```python
from build123d import *

# Parameters (mm, degrees)
EXTRUDE_1_DEPTH          = 9.45
EXTRUDE_1_DEPTH_BACK     = 9.45
EXTRUDE_2_DEPTH          = 14.45
EXTRUDE_2_DEPTH_BACK     = 14.45
CUT_EXTRUDE_1_DEPTH      = 24.45
CUT_EXTRUDE_1_DEPTH_BACK = 26.45
HOLE_WIZARD_M3_1_D       = 2.5
HOLE_WIZARD_M3_1_DEPTH   = 6.5
HOLE_WIZARD_M3_1_TIP     = 0.751075774


with BuildPart() as part:
    # Sketch 1 → Extrude 1 (new, two sides: drawn at the far end of the back side and taken through both)
    with BuildSketch(Plane(origin=(0, 0, 0), x_dir=(0, 0, -1), z_dir=(1, 0, 0)).offset(-EXTRUDE_1_DEPTH_BACK)):
        Polygon((-10, 7.500004795), (-10, 0.499995205), (-9.500004795, 0), (9.500004795, 0), (10, 0.499995205), (10, 7.500004795), (9.500004795, 8), (4.9, 8), (4.6, 7.7), (-4.6, 7.7), (-4.9, 8), (-9.500004795, 8), align=None)
    extrude(amount=EXTRUDE_1_DEPTH + EXTRUDE_1_DEPTH_BACK)

    # Sketch 2 → Extrude 2 (add, two sides: drawn at the far end of the back side and taken through both)
    with BuildSketch(Plane(origin=(0, 0, 0), x_dir=(0, 0, -1), z_dir=(1, 0, 0)).offset(-EXTRUDE_2_DEPTH_BACK)):
        Polygon((-9.8, 6.70000959), (-9.8, 0.599980104), (-9.200019896, 0), (9.200019896, 0), (9.8, 0.599980104), (9.8, 6.70000959), (8.80000959, 7.7), (-8.80000959, 7.7), align=None)
    extrude(amount=EXTRUDE_2_DEPTH + EXTRUDE_2_DEPTH_BACK)

    # Sketch 3 → Cut-Extrude 1 (cut, two sides: drawn at the far end of the back side and taken through both)
    with BuildSketch(Plane(origin=(0, 0, 0), x_dir=(0, 0, -1), z_dir=(1, 0, 0)).offset(-CUT_EXTRUDE_1_DEPTH_BACK)):
        with BuildLine():
            Line((-4.5, 4.199974593), (-4.5, 3.5583))
            ThreePointArc((-4.5, 3.5583), (-4.475010695, 3.475400506), (-4.408368985, 3.420122355))
            ThreePointArc((-4.408368985, 3.420122355), (-4.141124334, 3.252255308), (-3.93950231, 3.009464023))
            ThreePointArc((-3.93950231, 3.009464023), (-3.898814145, 2.964704671), (-3.843755349, 2.939655613))
            Line((-3.843755349, 2.939655613), (-3.466644651, 2.853644387))
            ThreePointArc((-3.466644651, 2.853644387), (-3.382732565, 2.800932608), (-3.35, 2.7074))
            Line((-3.35, 2.7074), (-3.35, 2.2926))
            ThreePointArc((-3.35, 2.2926), (-3.382732565, 2.199067392), (-3.466644651, 2.146355613))
            Line((-3.466644651, 2.146355613), (-3.843755349, 2.060344387))
            ThreePointArc((-3.843755349, 2.060344387), (-3.898814145, 2.035295329), (-3.93950231, 1.990535977))
            ThreePointArc((-3.93950231, 1.990535977), (-4.141123452, 1.74774336), (-4.408368985, 1.579877645))
            ThreePointArc((-4.408368985, 1.579877645), (-4.475010695, 1.524599494), (-4.5, 1.4417))
            Line((-4.5, 1.4417), (-4.5, -1.500004795))
            Line((-4.5, -1.500004795), (-4.000004795, -2))
            Line((-4.000004795, -2), (1.4, -2))
            ThreePointArc((1.4, -2), (1.8, -1.8), (2.2, -2))
            Line((2.2, -2), (4.000004795, -2))
            Line((4.000004795, -2), (4.5, -1.500004795))
            Line((4.5, -1.500004795), (4.5, 1.4417))
            ThreePointArc((4.5, 1.4417), (4.475010695, 1.524599494), (4.408368985, 1.579877645))
            ThreePointArc((4.408368985, 1.579877645), (4.141124334, 1.747744692), (3.93950231, 1.990535977))
            ThreePointArc((3.93950231, 1.990535977), (3.898814145, 2.035295329), (3.843755349, 2.060344387))
            Line((3.843755349, 2.060344387), (3.466644651, 2.146355613))
            ThreePointArc((3.466644651, 2.146355613), (3.382732565, 2.199067392), (3.35, 2.2926))
            Line((3.35, 2.2926), (3.35, 2.7074))
            ThreePointArc((3.35, 2.7074), (3.382732565, 2.800932608), (3.466644651, 2.853644387))
            Line((3.466644651, 2.853644387), (3.843755349, 2.939655613))
            ThreePointArc((3.843755349, 2.939655613), (3.898814145, 2.964704671), (3.93950231, 3.009464023))
            ThreePointArc((3.93950231, 3.009464023), (4.141123452, 3.25225664), (4.408368985, 3.420122355))
            ThreePointArc((4.408368985, 3.420122355), (4.475010695, 3.475400506), (4.5, 3.5583))
            Line((4.5, 3.5583), (4.5, 4.199974593))
            Line((4.5, 4.199974593), (4.199974593, 4.5))
            Line((4.199974593, 4.5), (-4.199974593, 4.5))
            Line((-4.199974593, 4.5), (-4.5, 4.199974593))
        make_face()
    extrude(amount=CUT_EXTRUDE_1_DEPTH + CUT_EXTRUDE_1_DEPTH_BACK, mode=Mode.SUBTRACT)

    # Sketch 12 → Cut-Revolve 6 (revolve, cut)
    with BuildSketch(Plane.XY.offset(5), mode=Mode.PRIVATE) as cut_revolve_6_sk:
        Polygon((-13.45, 6.2), (-13.45, 7), (-13.2605, 6.8105), (-9.45, 6.8105), (-9.097527661, 6.2), align=None)
    revolve(cut_revolve_6_sk.sketch.rotate(Axis((-9.097527661, 6.2, 5), (-1, 0, 0)), 270), axis=Axis((-9.097527661, 6.2, 5), (-1, 0, 0)), mode=Mode.SUBTRACT)

    # Hole Wizard M3 _1
    with Locations(Plane(origin=(0, 8, 0), x_dir=(1, 0, 0), z_dir=(0, 1, 0))):
        with Locations((5, -7.5), (-5, -7.5), (5, 7.5), (-5, 7.5)):
            Hole(HOLE_WIZARD_M3_1_D / 2, depth=HOLE_WIZARD_M3_1_DEPTH)
            with Locations((0, 0, -(HOLE_WIZARD_M3_1_DEPTH + HOLE_WIZARD_M3_1_TIP / 2))):  # 118° drill point
                Cone(0, HOLE_WIZARD_M3_1_D / 2, HOLE_WIZARD_M3_1_TIP, mode=Mode.SUBTRACT)


solid = part.part
```
Source: CAD feature listing. Evaluate the final solid. Frame: model axes, mm. A direction names the side the tool comes from. Give positions to 0.01 mm unless a question says otherwise; leave off trailing zeros. Order: outer loops, then holes, each group sorted by start corner. A loop starts at its lowest first (then second) coordinate and runs counter-clockwise, first axis right, second up.
(1) Pull-direction query (X, two-part tool) for faces 1 (the face through (5.27, 4.7, 8.72)), 2 (the face through (-14.45, 5, 0)), 3 (the face through (12, 4, -9.8)), 4 (the face through (4.78, 0.88, -7.51)); classes: +X half, -X half, draft (parallel to the pull), parting line (faces both ways), or undercut.
(2) Section query A-A (y = 5). Return the cut outline in (x, z), plus the area to 3 significant figures.
(3) Contact query for flat-ended pins moving along their axis: P1, Ø4, axis at x = -12, y = 3.5, coming from the +Z side; P2, Ø2, axis at x = 5, z = -7.5, coming from the +Y side; P3, Ø1.5, axis at x = 13, y = 3.5, coming from the -Z side. Output: stop coordinate, or through.
(4) Access query for faces 5 (the face through (-11.329, 5.829, 4.516)), 6 (the face through (12, 4, 9.8)), 7 (the face through (0, 4.5, 0)). Directions: +Z, -Z, +X, -X, +Y, -Y. A direction counts if a zero-diameter tool reaches every point of the face in a straight line with its end or side. Return the directions, or none.
(5) Section query B-B (z = 1.5). Return the cut outline in (x, y).
(6) Material intervals for line 1 along Z through (x, y) = (5, 7); line 2 along X through (y, z) = (3.5, 7.5); line 3 along Z through (x, y) = (-5, 3), sorted ascending.
Outcome:
1. face 1: undercut
1. face 2: -X half
1. face 3: draft
1. face 4: undercut
2. outline: (-14.45, -9.8) - (-9.45, -9.8) - (-9.45, -10) - (9.45, -10) - (9.45, -9.8) - (14.45, -9.8) - (14.45, 9.8) - (9.45, 9.8) - (9.45, 10) - (-9.45, 10) - (-9.45, 9.8) - (-14.45, 9.8) - close; hole circle Ø2.5 at (-5, -7.5); hole circle Ø2.5 at (-5, 7.5); hole circle Ø2.5 at (5, -7.5); hole circle Ø2.5 at (5, 7.5)
2. area: 554 mm2
3. P1: stops at z = 9.8
3. P2: stops at y = 1.35
3. P3: stops at z = -9.8
4. face 5: none
4. face 6: +Z, +X, +Y, -Y
4. face 7: +X, -X
5. outline: (-14.45, 4.5) - (14.45, 4.5) - (14.45, 7.7) - (-14.45, 7.7) - close
6. line 1: z = -10 to -8.75, -6.25 to 6.25, 8.75 to 10
6. line 2: x = -14.45 to -6.25, -3.75 to 3.75, 6.25 to 14.45
6. line 3: z = -10 to -8.75, -6.25 to -3.93, 3.93 to 6.25, 8.75 to 10
